```python
from build123d import *

# Parameters (mm, degrees)
F0_W     = 100
F0_H     = 80
F1_DEPTH = 30
F2_R     = 10.879287
F3_DEPTH = 25
F4_R     = 5


with BuildPart() as f1:
    # F0 (on Front) → F1 (new body)
    with BuildSketch(Plane.XZ):
        with Locations((50, 40)):
            Rectangle(F0_W, F0_H)
    extrude(amount=F1_DEPTH)

    # F2 (on face) → F3 (cut)
    with BuildSketch(Plane.XZ.offset(30)):
        with Locations((24.835449, 54.302912)):
            Circle(F2_R)
    extrude(amount=-F3_DEPTH, mode=Mode.SUBTRACT)

    # F4
    f4_edges = [f1.edges().sort_by_distance(p)[0] for p in [
        (0, -15, 80),
        (100, -15, 80),
        (100, -15, 0),
        (0, -15, 0),
    ]]
    fillet(f4_edges, radius=F4_R)


solid = f1.part
```
Input: part model. Units: mm. Frame: model coordinates. A direction names the side the tool comes from. Coordinates: 2 decimals unless noted, no trailing zeros. Write each loop counter-clockwise with the first axis right and the second up, starting at its lowest first coordinate (ties: lowest second). Pieces come first, ordered by that corner, then holes. Notation, with made-up numbers: (22.25, 8.25) - (49.25, 8.25) arc R19 ccw to (49.25, 42.25) - close; hole circle Ø2 at (63, -21). An arc over 180 degrees is marked (long way). Put each result on its own line as item: value. Start each with the question number.
1) Cut plane C-C (x = 26). Return the cut outline in (y, z).
2) Contact query for flat-ended pins moving along their axis: pin 1 (4 mm diameter, centred on x = 36, z = 31, fed in from +Y); pin 2 (6.5 mm diameter, centred on x = 26.5, z = 59.5, fed in from -Y). Output: stop coordinate, or through.
3) Reachability of faces 4 (the face through (29.856, -17.675, 44.651)), 5 (the face through (98, -15, 79)) from +Z, -Z, +X, -X, +Y, -Y: full face, straight path, thin tool, end or side. Return the list, or none.
4) Cut plane B-B (z = 59). Return the cut outline in (x, y), plus the area to 3 significant figures.
5) Cut plane A-A (y = -28). Return the cut outline in (x, z), plus the area to 3 significant figures.
6) Ray query, L1, parallel to Z at x = 34.5, y = -26.5; L2, parallel to Z at x = 32.5, y = -20.25; L3, parallel to X at y = -11.5, z = 51.5. Return the intervals inside material, ascending.
7) Mould query, pull axis X, two halves, no side actions, for faces 1 (the face through (25, -5, 54)), 2 (the face through (49, -15, 0)), 3 (the face through (0, -15, 40)). Classes: pulls with the +X half, pulls with the -X half, needs draft (parallel to the pull), parting line crosses it, or undercut.
Resolved:
1. outline: (-30, 0) - (0, 0) - (0, 80) - (-30, 80) - (-30, 65.12) - (-5, 65.12) - (-5, 43.49) - (-30, 43.49) - close
2. pin 1: stops at y = 0
2. pin 2: stops at y = -5
3. face 4: -Y
3. face 5: +Z, +X, +Y, -Y
4. outline: (0, -30) - (15.02, -30) - (15.02, -5) - (34.65, -5) - (34.65, -30) - (100, -30) - (100, 0) - (0, 0) - close
4. area: 2,510 mm2
5. outline: (0, 5) arc R5 ccw to (5, 0) - (95, 0) arc R5 ccw to (100, 5) - (100, 75) arc R5 ccw to (95, 80) - (5, 80) arc R5 ccw to (0, 75) - close; hole circle Ø21.76 at (24.84, 54.3)
5. area: 7,610 mm2
6. L1: z = 0 to 49.31, 59.3 to 80
6. L2: z = 0 to 46.58, 62.02 to 80
6. L3: x = 0 to 14.32, 35.35 to 100
7. face 1: undercut
7. face 2: needs draft
7. face 3: pulls with the -X half
